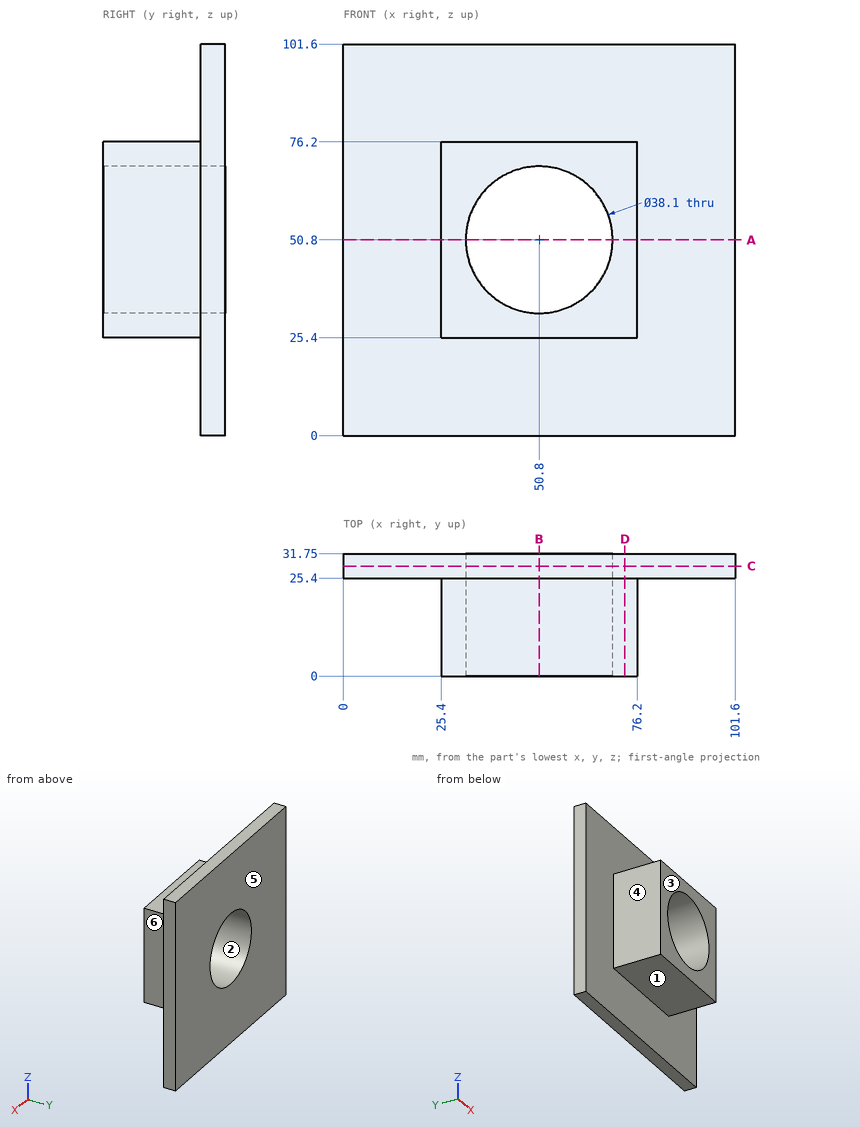
Print and shaded views of the part. All mm, measured from the part's lowest x, y and z. A direction names the side the tool comes from. Round coordinates to 2 decimals unless told otherwise and drop trailing zeros. Order: outer loops, then holes, each group sorted by start corner. A loop starts at its lowest first (then second) coordinate and runs counter-clockwise, first axis right, second up. Notation, with made-up numbers: (-31, -36.75) - (2, -36.75) arc R32 cw to (2, -10.75) - close; hole circle Ø2 at (-10, 72). An arc over 180 degrees is marked (long way). Use a Markdown table: item, result.
1) Wall check: L1, parallel to Z at x = 50.8, y = 24; L2, parallel to X at y = 22, z = 50; L3, parallel to Y at x = 50.5, z = 7. Give the ranges that are in metal, low to high.
Recorded:
| item | result |
|---|---|
| L1 | z = 25.4 to 31.75, 69.85 to 76.2 |
| L2 | x = 25.4 to 31.77, 69.83 to 76.2 |
| L3 | y = 25.4 to 31.75 |
2) Saw through at A-A on z = 50.8. Write the cut outline in (x, y).
Recorded:
| item | result |
|---|---|
| outline | (0, 25.4) - (25.4, 25.4) - (25.4, 0) - (31.75, 0) - (31.75, 31.75) - (0, 31.75) - close; (69.85, 0) - (76.2, 0) - (76.2, 25.4) - (101.6, 25.4) - (101.6, 31.75) - (69.85, 31.75) - close |
3) Saw through at B-B on x = 50.8. Write the cut outline in (y, z), and give its area (3 significant figures).
Recorded:
| item | result |
|---|---|
| outline | (0, 25.4) - (25.4, 25.4) - (25.4, 0) - (31.75, 0) - (31.75, 31.75) - (0, 31.75) - close; (0, 69.85) - (31.75, 69.85) - (31.75, 101.6) - (25.4, 101.6) - (25.4, 76.2) - (0, 76.2) - close |
| area | 726 mm² |
4) Tool access for the marked faces 4, 5 and 6: list every direction of +Z, -Z, +X, -X, +Y, -Y with a clear straight run to the whole face (end or side of a thin tool).
Recorded:
| item | result |
|---|---|
| face 4 | +Z, -Z, -X, -Y |
| face 5 | +Z, -Z, +X, -X, +Y |
| face 6 | +Z, -Z, +X, -Y |
5) Saw through at C-C on y = 28.5. Write the cut outline in (x, z), and give its area (3 significant figures).
Recorded:
| item | result |
|---|---|
| outline | (0, 0) - (101.6, 0) - (101.6, 101.6) - (0, 101.6) - close; hole circle Ø38.1 at (50.8, 50.8) |
| area | 9,180 mm² |
6) Flat gauge pins, fed straight in: pin 1 Ø12.5 at (x, y) = (54.5, 16.5) entering from +Z; pin 2 Ø2 at (x, y) = (55, 22) entering from -Z; pin 3 Ø7.5 at (y, z) = (15.5, 40) entering from -X. Where does each tip first touch, or does it go through?
Recorded:
| item | result |
|---|---|
| pin 1 | stops at z = 76.2 |
| pin 2 | stops at z = 25.4 |
| pin 3 | stops at x = 25.4 |
7) Pull direction Z, two halves, no side cores. Call the marked faces 1, 2 and 3: pulls with the +Z half, pulls with the -Z half, needs draft (parallel to the pull), parting line crosses it, or undercut.
Recorded:
| item | result |
|---|---|
| face 1 | pulls with the -Z half |
| face 2 | undercut |
| face 3 | needs draft |
8) Saw through at D-D on x = 73. Write the cut outline in (y, z).
Recorded:
| item | result |
|---|---|
| outline | (0, 25.4) - (25.4, 25.4) - (25.4, 0) - (31.75, 0) - (31.75, 101.6) - (25.4, 101.6) - (25.4, 76.2) - (0, 76.2) - close |
